Here's how the part is built. I have some questions about the finished solid (model axes, mm). A direction names the side the tool comes from. Round coordinates to 2 decimals unless told otherwise and drop trailing zeros. Write each loop counter-clockwise with the first axis right and the second up, starting at its lowest first coordinate (ties: lowest second). Pieces come first, ordered by that corner, then holes. Notation, with made-up numbers: (-39.5, 18) -> (9.5, 18) arc R21 cw to (9.5, 52) -> close; hole circle Ø11 at (5.25, 77). An arc over 180 degrees is marked (long way). Put each result on its own line as item: value. Start each with the question number.
1) I want a section at D-D, the plane z = 42. List the corners of the cut face in (x, y) for me, then the cut area to 3 significant figures.
2) Which directions (+Z, -Z, +X, -X, +Y, -Y) give clear straight access to the entire face, cutting with the end or side of a thin tool? Please do faces 4 (the flat face through (-1, 0, -25)), 5 (the flat face through (-1, 0, 35)), 6 (the cylindrical face through (87.372, 38.375, 12.878)), 7 (the flat face through (10, -12.7, -10)), 8 (the flat face through (-1, 39.824, 15)).
3) I want a section at A-A, the plane x = 0. List the corners of the cut face in (y, z) for me, then the cut area to 3 significant figures.
4) We'd pull the mould along X, two halves only. Please class faces 1 (the flat face through (-88.9, 14, 13)), 2 (the flat face through (88.9, 14, 13)), 3 (the cylindrical face through (21.579, -19.139, 6.796)): released by +X, released by -X, zero draft, split by the parting line, or undercut.
5) Will these pins go through, and if not, where does the flat tip stop? P1, Ø12, axis at x = 46.5, y = 11, coming from the -Z side; P2, Ø13.5, axis at x = 5.5, z = -10, coming from the -Y side; P3, Ø7.5, axis at x = -19.5, z = 44, coming from the +Y side.
6) I want a section at B-B, the plane y = 20. List the corners of the cut face in (x, z) for me.
7) If I drill on line 1 along Z through (x, y) = (0, -16); line 2 along Y through (x, z) = (43.5, -12.5); line 3 along X through (y, z) = (18.5, 17.5), over which ranges is the centre line in solid material (lowest first)? Write a range as [from, to].
8) I want a section at C-C, the plane x = -35.5. List the corners of the cut face in (y, z) for me.
from build123d import *

# Parameters (mm, degrees)
F0_R      = 50.8
F0_R_2    = 12.7
F1_DEPTH  = 25.4
F2_W      = 177.8
F2_H      = 50.8
F3_DEPTH  = 25.4
F5_R      = 22.6237609961
F6_DEPTH  = 12.7
F7_R      = 10.2865280917
F8_DEPTH  = 25.4
F9_R      = 5.08
F11_R     = 12.7
F12_DEPTH = 76.2


# Not quite as in the source:
# - a feature names something its author has since deleted; it is built from what else it names


with BuildPart() as f1:
    # F0 (on Front) → F1 (new body)
    with BuildSketch(Plane.XZ):
        Circle(F0_R)
        Circle(F0_R_2, mode=Mode.SUBTRACT)
    extrude(amount=F1_DEPTH)

    # F2 (on Top) → F3 (join)
    with BuildSketch(Plane.XY):
        with Locations((0, 14.4235261992)):
            Rectangle(F2_W, F2_H)
    extrude(amount=F3_DEPTH)

    # F4: union 

    # F5 (on face) → F6 (cut)
    with BuildSketch(Plane.XZ.offset(25.4)):
        Circle(F5_R)
    extrude(amount=-F6_DEPTH, mode=Mode.SUBTRACT)

    # F7 (on face) → F8 (cut)
    with BuildSketch(Plane.XY.offset(25.4)):
        with Locations((-66.7031380003, 14.4235261992)):
            Circle(F7_R)
        with Locations((66.7031380003, 14.4235261992)):
            Circle(F7_R)
    extrude(amount=-F8_DEPTH, mode=Mode.SUBTRACT)

    # F9
    f9_edges = [f1.edges().sort_by_distance(p)[0] for p in [
        (88.9, 39.823526, 12.7),
        (-88.9, 39.823526, 12.7),
        (-88.9, -10.976474, 12.7),
        (88.9, -10.976474, 12.7),
    ]]
    fillet(f9_edges, radius=F9_R)

    # F11 (on face) → F12 (cut)
    with BuildSketch(Plane.XZ.offset(25.4)):
        Circle(F11_R)
    extrude(amount=-F12_DEPTH, mode=Mode.SUBTRACT)


solid = f1.part
Findings:
1. outline: (-28.58, -25.4) -> (28.58, -25.4) -> (28.58, 0) -> (-28.58, 0) -> close
1. area: 1,450 mm2
2. face 4: -Z, +X, -X, +Y
2. face 5: +Z, +X, -X, +Y
2. face 6: +Z, -Z, +X, +Y
2. face 7: -Y
2. face 8: +Z, -Z, +X, -X, +Y
3. outline: (-25.4, -50.8) -> (0, -50.8) -> (0, -12.7) -> (-12.7, -12.7) -> (-12.7, -22.62) -> (-25.4, -22.62) -> close; (-25.4, 22.62) -> (-12.7, 22.62) -> (-12.7, 12.7) -> (39.82, 12.7) -> (39.82, 25.4) -> (0, 25.4) -> (0, 50.8) -> (-25.4, 50.8) -> close
3. area: 2,190 mm2
4. face 1: released by -X
4. face 2: released by +X
4. face 3: undercut
5. P1: stops at z = 0
5. P2: stops at y = -12.7
5. P3: stops at y = 0
6. outline: (-88.9, 0) -> (-75.35, 0) -> (-75.35, 25.4) -> (-88.9, 25.4) -> close; (-58.06, 0) -> (-12.7, 0) arc R12.7 cw to (12.7, 0) -> (58.06, 0) -> (58.06, 25.4) -> (-58.06, 25.4) -> close; (75.35, 0) -> (88.9, 0) -> (88.9, 25.4) -> (75.35, 25.4) -> close
7. line 1: z = [-50.8, -22.62], [22.62, 50.8]
7. line 2: y = [-25.4, 0]
7. line 3: x = [-88.9, -76.15], [-57.26, 57.26], [76.15, 88.9]
8. outline: (-25.4, -36.34) -> (0, -36.34) -> (0, 0) -> (39.82, 0) -> (39.82, 25.4) -> (0, 25.4) -> (0, 36.34) -> (-25.4, 36.34) -> close
